Geometry check sheet. Reference: the model listing, model coordinates, mm. Give positions to 0.01 mm unless a question says otherwise; leave off trailing zeros. Order: outer loops, then holes, each group sorted by start corner. A loop starts at its lowest first (then second) coordinate and runs counter-clockwise, first axis right, second up. Notation, with made-up numbers: M -17.5,34.5 L 9.5,34.5 A14 ccw 9.5,60.5 Z; hole C 9.5,64.25 d8. An arc over 180 degrees is marked long. Answer as CSV lines item,"result".
from build123d import *

# Parameters (mm, degrees)
SKETCH1_W           = 25
SKETCH1_H           = 10
SKETCH1_R           = 2.404163056
SKETCH1_R_2         = 2.333452378
SKETCH1_R_3         = 2.474873734
BOSS_EXTRUDE1_DEPTH = 10
CHAMFER1_SIZE       = 0.5


with BuildPart() as part:
    # Sketch1 → Boss-Extrude1 (new body)
    with BuildSketch(Plane.XY):
        Rectangle(SKETCH1_W, SKETCH1_H)
        Circle(SKETCH1_R, mode=Mode.SUBTRACT)
        with Locations((-8, 0)):
            Circle(SKETCH1_R_2, mode=Mode.SUBTRACT)
        with Locations((8, 0)):
            Circle(SKETCH1_R_3, mode=Mode.SUBTRACT)
    extrude(amount=BOSS_EXTRUDE1_DEPTH)

    # Chamfer1
    chamfer1_edges = [part.edges().sort_by_distance(p)[0] for p in [
        (-2.404163056, 0, 10),
        (5.525126266, 0, 10),
        (-10.333452378, 0, 10),
    ]]
    chamfer(chamfer1_edges, length=CHAMFER1_SIZE)


solid = part.part
(1) Section check D-D on x = -8. Enter the section's corners in (y, z).
The answers:
outline,"M -5,0 L -2.33,0 L -2.33,9.5 L -2.83,10 L -5,10 Z; M 2.33,0 L 5,0 L 5,10 L 2.83,10 L 2.33,9.5 Z"
(2) Material ranges on line 1 (X direction, y = 0.25, z = 6.5); line 2 (X direction, y = -1.5, z = 2.5); line 3 (Y direction, x = -10, z = 3.5), recorded low to high.
The answers:
line 1,"x = -12.5 to -10.32, -5.68 to -2.39, 2.39 to 5.54, 10.46 to 12.5"
line 2,"x = -12.5 to -9.79, -6.21 to -1.88, 1.88 to 6.03, 9.97 to 12.5"
line 3,"y = -5 to -1.2, 1.2 to 5"
(3) Section check C-C on z = 2. Enter the section's corners in (x, y), then the cut area to 3 significant figures.
The answers:
outline,"M -12.5,-5 L 12.5,-5 L 12.5,5 L -12.5,5 Z; hole C -8,0 d4.67; hole C 0,0 d4.81; hole C 8,0 d4.95"
area,"195 mm2"
(4) Gauge pin test, flat end, axial feed: P1, Ø3, axis at x = 8, y = 0, coming from the -Z side. Record the tip position at first contact, or that the pin passes through.
The answers:
P1,"passes through"
(5) Draft check along Y on faces 1 (the face through (-3, -1, 10)), 2 (the face through (0, 5, 5)), 3 (the face through (5.528, 0.109, 4.684)). Enter one of: +Y half, -Y half, draft (parallel to the pull), parting line (faces both ways), or undercut.
The answers:
face 1,"draft"
face 2,"+Y half"
face 3,"undercut"
(6) Section check A-A on y = 0. Enter the section's corners in (x, z).
The answers:
outline,"M -12.5,0 L -10.33,0 L -10.33,9.5 L -10.83,10 L -12.5,10 Z; M -5.67,0 L -2.4,0 L -2.4,9.5 L -2.9,10 L -5.17,10 L -5.67,9.5 Z; M 2.4,0 L 5.53,0 L 5.53,9.5 L 5.03,10 L 2.9,10 L 2.4,9.5 Z; M 10.47,0 L 12.5,0 L 12.5,10 L 10.97,10 L 10.47,9.5 Z"
(7) Section check B-B on x = 8. Enter the section's corners in (y, z).
The answers:
outline,"M -5,0 L -2.47,0 L -2.47,9.5 L -2.97,10 L -5,10 Z; M 2.47,0 L 5,0 L 5,10 L 2.97,10 L 2.47,9.5 Z"
